Job drawing, mm, ordinate dimensions from the low corner. One solid piece. A direction names the side the tool comes from. Round coordinates to 2 decimals unless told otherwise and drop trailing zeros. Write each loop counter-clockwise with the first axis right and the second up, starting at its lowest first coordinate (ties: lowest second). Pieces come first, ordered by that corner, then holes. Notation, with made-up numbers: M 73.5,82.5 L 106.5,82.5 A14 cw 106.5,92.5 Z; hole C 72.5,-8.75 d3. An arc over 180 degrees is marked long. One line per item, written item: value. Start each with the question number.
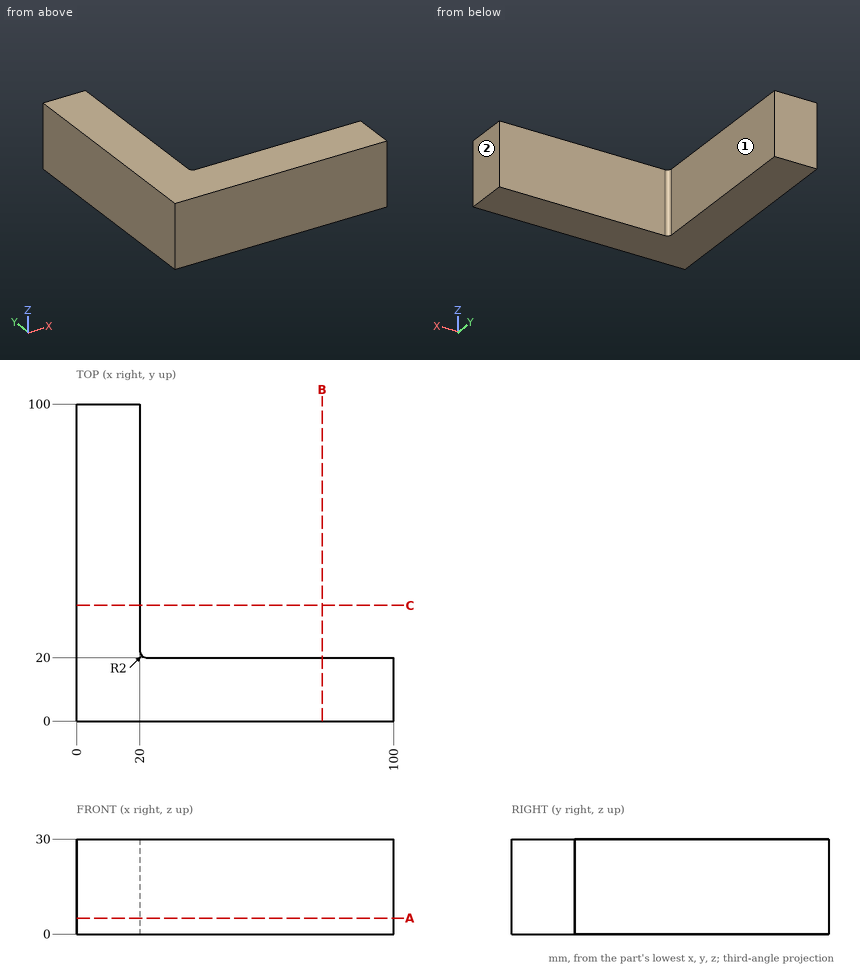
Item 1: Which spindle directions (+Z, -Z, +X, -X, +Y, -Y) get a long thin tool onto all of the face, cutting with end or side? Do the marked faces 1 and 2. Say none if no direction does.
Item 2: Cut at B-B, the plane x = 77.5. Write the cut outline in (y, z).
Item 3: Drop flat-ended pins along their axis: pin 1 (3 mm diameter, centred on x = 39.5, z = 3, fed in from +Y); pin 2 (15 mm diameter, centred on y = 64.5, z = 16.5, fed in from +X). Give the stop position or say it passes through.
Item 4: Cut at A-A, the plane z = 5. Write the cut outline in (x, y), plus the area to 3 significant figures.
Item 5: Drill centre lines: line 1 (Y direction, x = 61, z = 6.5); line 2 (Y direction, x = 21.5, z = 4.75). Where is each one in solid material? Low to high.
Computed values:
1. face 1: +Z, -Z, +X, +Y
1. face 2: +Z, -Z, +X, +Y, -Y
2. outline: M 0,0 L 20,0 L 20,30 L 0,30 Z
3. pin 1: stops at y = 20
3. pin 2: stops at x = 20
4. outline: M 0,0 L 100,0 L 100,20 L 22,20 A2 cw 20,22 L 20,100 L 0,100 Z
4. area: 3,600 mm2
5. line 1: y = 0 to 20
5. line 2: y = 0 to 20.06
